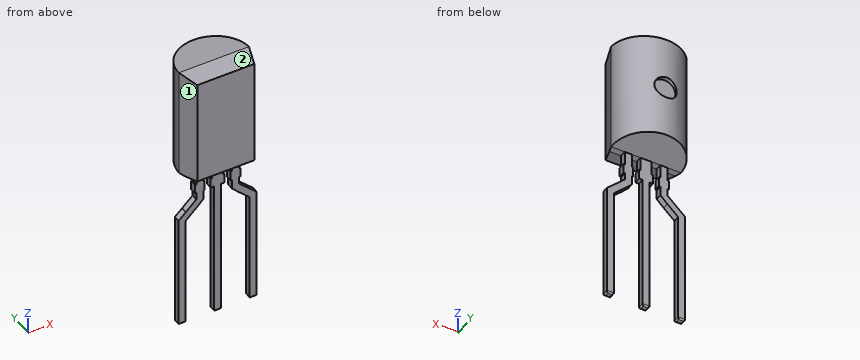
from build123d import *

# Parameters (mm, degrees)
BOSS_EXTRUDE2_DEPTH = 8
BOSS_EXTRUDE3_DEPTH = 0.225
BOSS_EXTRUDE4_DEPTH = 0.225
BOSS_EXTRUDE7_DEPTH = 0.225
BOSS_EXTRUDE8_DEPTH = 0.225
CUT_EXTRUDE1_DEPTH  = 5
CUT_EXTRUDE2_DEPTH  = 5
CUT_EXTRUDE3_DEPTH  = 5
CUT_EXTRUDE7_DEPTH  = 5
FILLET2_R           = 0.1
SKETCH13_R          = 0.8
CUT_EXTRUDE8_DEPTH  = 0.3


with BuildPart() as part:
    # Sketch1 → Boss-Extrude2 (new body)
    with BuildSketch(Plane.XY):
        with BuildLine():
            Line((-2.036541185, -1.45), (2.036541185, -1.45))
            Line((2.036541185, -1.45), (2.5, 0))
            ThreePointArc((2.5, 0), (0, 2.5), (-2.5, 0))
            Line((-2.5, 0), (-2.036541185, -1.45))
        make_face()
    extrude(amount=BOSS_EXTRUDE2_DEPTH)

    # Sketch3 → Boss-Extrude3 (add)
    with BuildSketch(Plane(origin=(0, -0.225, 0), x_dir=(1, 0, 0), z_dir=(0, 1, 0))):
        Polygon((-0.4, 0), (0.4, 0), (0.4, 1), (0.5, 1), (0.5, 1.7), (0.25, 1.7), (0.25, 11.7), (-0.25, 11.7), (-0.25, 1.7), (-0.5, 1.7), (-0.5, 1), (-0.4, 1), align=None)
    extrude(amount=BOSS_EXTRUDE3_DEPTH)

    # Sketch3<3> → Boss-Extrude4 (add)
    with BuildSketch(Plane(origin=(0, -0.225, 0), x_dir=(1, 0, 0), z_dir=(0, 1, 0))):
        Polygon((-0.4, 0), (0.4, 0), (0.4, 1), (0.5, 1), (0.5, 1.7), (0.25, 1.7), (0.25, 11.7), (-0.25, 11.7), (-0.25, 1.7), (-0.5, 1.7), (-0.5, 1), (-0.4, 1), align=None)
    extrude(amount=-BOSS_EXTRUDE4_DEPTH)

    # Sketch7 → Boss-Extrude7 (add)
    with BuildSketch(Plane(origin=(0, -0.225, 0), x_dir=(1, 0, 0), z_dir=(0, 1, 0))):
        Polygon((1.02, 1), (1.02, 0), (1.27, 0), (1.52, 0), (1.52, 1), (1.62, 1), (1.62, 1.7), (1.52, 1.7), (1.52, 2.211954512), (2.250085443, 2.896837591), (2.249444332, 2.897521015), (2.250813973, 2.897521015), (2.29, 2.934280887), (2.79, 3.403323987), (2.79, 4.08889049), (2.79, 11.7), (2.29, 11.7), (2.29, 3.61984739), (1.52, 2.897521015), (1.02, 2.397521015), (1.02, 2.211954512), (1.02, 1.7), (0.92, 1.7), (0.92, 1), align=None)
    boss_extrude7 = extrude(amount=BOSS_EXTRUDE7_DEPTH)

    # Sketch7<7> → Boss-Extrude8 (add)
    with BuildSketch(Plane(origin=(0, -0.225, 0), x_dir=(1, 0, 0), z_dir=(0, 1, 0))):
        Polygon((1.02, 1), (1.02, 0), (1.27, 0), (1.52, 0), (1.52, 1), (1.62, 1), (1.62, 1.7), (1.52, 1.7), (1.52, 2.211954512), (2.250085443, 2.896837591), (2.249444332, 2.897521015), (2.250813973, 2.897521015), (2.29, 2.934280887), (2.79, 3.403323987), (2.79, 4.08889049), (2.79, 11.7), (2.29, 11.7), (2.29, 3.61984739), (1.52, 2.897521015), (1.02, 2.397521015), (1.02, 2.211954512), (1.02, 1.7), (0.92, 1.7), (0.92, 1), align=None)
    boss_extrude8 = extrude(amount=-BOSS_EXTRUDE8_DEPTH)

    # Mirror2: Boss-Extrude7, Boss-Extrude8 across plane
    add(boss_extrude7.mirror(Plane(origin=(0, 0, 0), x_dir=(0, 0, 1), z_dir=(1, 0, 0))))
    add(boss_extrude8.mirror(Plane(origin=(0, 0, 0), x_dir=(0, 0, 1), z_dir=(1, 0, 0))))

    # Sketch9 → Cut-Extrude1 (cut)
    with BuildSketch(Plane(origin=(2.5, 0, 0), x_dir=(0, 0, -1), z_dir=(1, 0, 0))):
        Polygon((-8, 0), (-7.8, 2.5), (-8, 2.5), align=None)
    extrude(amount=-CUT_EXTRUDE1_DEPTH, mode=Mode.SUBTRACT)

    # Sketch10 → Cut-Extrude2 (cut)
    with BuildSketch(Plane(origin=(2.5, 0, 0), x_dir=(0, 0, -1), z_dir=(1, 0, 0))):
        Polygon((-8, 0), (-8, -1.45), (-7.85, -1.45), align=None)
    extrude(amount=-CUT_EXTRUDE2_DEPTH, mode=Mode.SUBTRACT)

    # Sketch11 → Cut-Extrude3 (cut)
    with BuildSketch(Plane(origin=(2.5, 0, 0), x_dir=(0, 0, -1), z_dir=(1, 0, 0))):
        Polygon((-0.2, 2.5), (0, 0), (0, 2.5), align=None)
    extrude(amount=-CUT_EXTRUDE3_DEPTH, mode=Mode.SUBTRACT)

    # Sketch12 → Cut-Extrude7 (cut)
    with BuildSketch(Plane(origin=(2.5, 0, 0), x_dir=(0, 0, -1), z_dir=(1, 0, 0))):
        Polygon((0, -0.45), (0, -1.45), (-0.15, -1.45), align=None)
    extrude(amount=-CUT_EXTRUDE7_DEPTH, mode=Mode.SUBTRACT)

    # Fillet2
    fillet2_edges = [part.edges().sort_by_distance(p)[0] for p in [
        (2.54, -0.45, -11.7),
        (0, 0, -11.7),
        (0.25, -0.225, -11.7),
        (-2.29, -0.225, -11.7),
        (-2.79, -0.225, -11.7),
        (-0.25, -0.225, -11.7),
        (-2.54, 0, -11.7),
        (-2.54, -0.45, -11.7),
        (0, -0.45, -11.7),
        (2.54, 0, -11.7),
        (2.79, -0.225, -11.7),
        (2.29, -0.225, -11.7),
    ]]
    fillet(fillet2_edges, radius=FILLET2_R)

    # Sketch13 → Cut-Extrude8 (cut)
    with BuildSketch(Plane(origin=(0, 2.5, 0), x_dir=(1, 0, 0), z_dir=(0, 1, 0))):
        with Locations((0, -4)):
            Circle(SKETCH13_R)
    extrude(amount=-CUT_EXTRUDE8_DEPTH, mode=Mode.SUBTRACT)


solid = part.part
The listing builds one solid part. Answer for the finished solid, in the listing's coordinates (mm). Face numbers are marked on the shaded views. A direction names the side the tool comes from. Coordinates: 2 decimals unless noted, no trailing zeros. Write each loop counter-clockwise with the first axis right and the second up, starting at its lowest first coordinate (ties: lowest second). Pieces come first, ordered by that corner, then holes. Notation, with made-up numbers: M -22,89.5 L -5,89.5 A25 cw -5,123.5 Z; hole C -28.5,4.25 d10. An arc over 180 degrees is marked long. Put each result on its own line as item: value. Start each with the question number.
1. A cutting plane is placed at D-D on y = 0.5. Write down the section's boundary in (x, z).
2. A cutting plane is placed at A-A on z = -9.25. Write down the section's boundary in (x, y).
3. Flat-ended cylindrical pins translate along their axes: P1, Ø2, axis at x = 1.5, z = -8.5, coming from the +Y side; P2, Ø1.5, axis at x = -0.5, y = 2, coming from the -Z side; P3, Ø0.6, axis at x = 2, z = -3.5, coming from the -Y side. Find the tip coordinate at first contact, or state that the pin passes through.
4. A cutting plane is placed at B-B on x = 1.3. Write down the section's boundary in (y, z), then the cut area to 3 significant figures.
5. Consider line 1 (X direction, y = -0.4, z = -4); line 2 (Y direction, x = 0.1, z = -2.75); line 3 (Y direction, x = -1.1, z = 5.75) (3 decimals). Determine where each line is inside the solid, lowest interval first. Write a range as from..to.
6. Which of the six approach directions +Z, -Z, +X, -X, +Y, -Y give full straight-line access (tool end or side, diameter ignored) to the marked faces 1 and 2?
7. A cutting plane is placed at C-C on z = 4. Write down the section's boundary in (x, y), then the cut area to 3 significant figures.
Resolved:
1. outline: M -2.45,0.04 L 2.45,0.04 L 2.45,7.96 L -2.45,7.96 Z
2. outline: M -2.79,-0.45 L -2.29,-0.45 L -2.29,0 L -2.79,0 Z; M -0.25,-0.45 L 0.25,-0.45 L 0.25,0 L -0.25,0 Z; M 2.29,-0.45 L 2.79,-0.45 L 2.79,0 L 2.29,0 Z
3. P1: stops at y = 0
3. P2: stops at z = 0.1
3. P3: stops at y = -0.45
4. outline: M -1.45,0.15 L -0.45,0 L -0.45,-2.68 L 0,-2.68 L 0,0 L 2.14,0.17 L 2.14,7.83 L 0,8 L -1.45,7.85 Z
4. area: 29.3 mm2
5. line 1: x = -2.79..-2.29, -0.25..0.25, 2.29..2.79
5. line 2: y = -0.45..0
5. line 3: y = -1.45..2.245
6. face 1: +Z, -X, -Y
6. face 2: +Z, +X, -X, -Y
7. outline: M -2.5,0 L -2.04,-1.45 L 2.04,-1.45 L 2.5,0 A2.5 ccw 0.8,2.37 L 0.8,2.2 L -0.8,2.2 L -0.8,2.37 A2.5 ccw Z
7. area: 16.0 mm2
